Could you check a few things on this model? Use its own coordinates, in mm. Coordinates: 2 decimals unless noted, no trailing zeros. Write each loop counter-clockwise with the first axis right and the second up, starting at its lowest first coordinate (ties: lowest second). Pieces come first, ordered by that corner, then holes.
Item 1: I want a section at C-C on z = 12.5. Please give me the cut outline in (x, y), then the cut area to 3 significant figures.
Item 2: I want a section at A-A on z = -19. Please give me the cut outline in (x, y), then the cut area to 3 significant figures.
Item 3: Thinking about a two-plate mould opening in X: for faces 1 (the flat face through (-75.394, -56, 1)), 2 (the flat face through (-66, -56, 42.467)), 3 (the flat face through (75.394, -56, -1)), 4 (the cylindrical face through (1.403, -55.804, -24.914)), which applies, +X half, -X half, draft (parallel to the pull), parting line (faces both ways), or undercut?
Item 4: For P1, Ø2, axis at x = -10.5, y = -66, coming from the +Z side; P2, Ø12, axis at x = -0.5, y = -62.5, coming from the +Z side, each with a flat end and sliding along its axis, tell me the tip position at first contact or that it passes through.
Item 5: I want a section at B-B on y = -12. Please give me the cut outline in (x, z), then the cut area to 3 significant figures.
Item 6: If I drill on probe 1 along X at (y, z) = (-107, 31); probe 2 along X at (y, z) = (-29, -3.5); probe 3 along Z at (x, y) = (20, -9), over which ranges is the centre line in solid material (lowest first)?
Item 7: I want a section at D-D on x = -53.5. Please give me the cut outline in (y, z), then the cut area to 3 significant figures.
from build123d import *

# Parameters (mm, degrees)
F1_DEPTH = 113.19281


with BuildPart() as f1:
    # F0 (on Front) → F1 (new body)
    with BuildSketch(Plane.XZ):
        with BuildLine():
            Line((75.394042, -42.466845), (75.394042, 42.466845))
            Line((75.394042, 42.466845), (56.622468, 42.466845))
            ThreePointArc((56.622468, 42.466845), (4e-06, -24.931278), (-56.62246, 42.466845))
            Line((-56.62246, 42.466845), (-75.394042, 42.466845))
            Line((-75.394042, 42.466845), (-75.394042, -42.466845))
            Line((-75.394042, -42.466845), (75.394042, -42.466845))
        make_face()
    extrude(amount=F1_DEPTH)


solid = f1.part
Response values:
1. outline: (-75.39, -113.19) - (-53.87, -113.19) - (-53.87, 0) - (-75.39, 0) - close; (53.87, -113.19) - (75.39, -113.19) - (75.39, 0) - (53.87, 0) - close
1. area: 4,870 mm2
2. outline: (-75.39, -113.19) - (-25.43, -113.19) - (-25.43, 0) - (-75.39, 0) - close; (25.43, -113.19) - (75.39, -113.19) - (75.39, 0) - (25.43, 0) - close
2. area: 11,300 mm2
3. face 1: -X half
3. face 2: draft
3. face 3: +X half
3. face 4: undercut
4. P1: stops at z = -23.77
4. P2: stops at z = -24.56
5. outline: (-75.39, -42.47) - (75.39, -42.47) - (75.39, 42.47) - (56.62, 42.47) arc R57.48 cw (long way) to (-56.62, 42.47) - (-75.39, 42.47) - close
5. area: 6,480 mm2
6. probe 1: x = -75.39 to -57.46, 57.46 to 75.39
6. probe 2: x = -75.39 to -44.77, 44.77 to 75.39
6. probe 3: z = -42.47 to -21.34
7. outline: (-113.19, -42.47) - (0, -42.47) - (0, 11.53) - (-113.19, 11.53) - close
7. area: 6,110 mm2
